```python
from build123d import *

# Parameters (mm, degrees)
SALIENTE_EXTRUIR1_DEPTH = 7
CROQUIS2_R              = 2.5
CORTAR_EXTRUIR1_DEPTH   = 8
CROQUIS3_R              = 1.5
CORTAR_EXTRUIR2_DEPTH   = 8
CROQUIS4_R              = 11
CROQUIS4_R_2            = 2.5
SALIENTE_EXTRUIR2_DEPTH = 2
REDONDEO1_R             = 0.1
REDONDEO3_R             = 0.25


with BuildPart() as part:
    # Croquis1 → Saliente-Extruir1 (new body)
    with BuildSketch(Plane(origin=(0, 0, 0), x_dir=(1, 0, 0), z_dir=(0, 1, 0))):
        Polygon((0, 32.526911935), (2.473088065, 35), (32.526911935, 35), (35, 32.526911935), (35, 2.473088065), (32.526911935, 0), (2.473088065, 0), (0, 2.473088065), align=None)
    extrude(amount=SALIENTE_EXTRUIR1_DEPTH)

    # Croquis2 → Cortar-Extruir1 (cut, through all)
    with BuildSketch(Plane(origin=(0, 7, 0), x_dir=(1, 0, 0), z_dir=(0, 1, 0))):
        with Locations((17.5, 17.5)):
            Circle(CROQUIS2_R)
    extrude(amount=-CORTAR_EXTRUIR1_DEPTH, mode=Mode.SUBTRACT)

    # Croquis3 → Cortar-Extruir2 (cut, through all)
    with BuildSketch(Plane(origin=(0, 7, 0), x_dir=(1, 0, 0), z_dir=(0, 1, 0))):
        with Locations((4.5, 30.5)):
            Circle(CROQUIS3_R)
        with Locations((30.5, 30.5)):
            Circle(CROQUIS3_R)
        with Locations((30.5, 4.5)):
            Circle(CROQUIS3_R)
        with Locations((4.5, 4.5)):
            Circle(CROQUIS3_R)
    extrude(amount=-CORTAR_EXTRUIR2_DEPTH, mode=Mode.SUBTRACT)

    # Croquis4 → Saliente-Extruir2 (add)
    with BuildSketch(Plane(origin=(0, 7, 0), x_dir=(1, 0, 0), z_dir=(0, 1, 0))):
        with Locations((17.5, 17.5)):
            Circle(CROQUIS4_R)
        with Locations((17.5, 17.5)):
            Circle(CROQUIS4_R_2, mode=Mode.SUBTRACT)
    extrude(amount=SALIENTE_EXTRUIR2_DEPTH)

    # Redondeo1
    redondeo1_edges = [part.edges().sort_by_distance(p)[0] for p in [
        (6.5, 9, -17.5),
    ]]
    fillet(redondeo1_edges, radius=REDONDEO1_R)

    # Redondeo3
    redondeo3_edges = [part.edges().sort_by_distance(p)[0] for p in [
        (17.5, 7, 0),
        (33.763455967, 7, -1.236544033),
        (35, 7, -17.5),
        (33.763455967, 7, -33.763455967),
        (17.5, 7, -35),
        (1.236544033, 7, -33.763455967),
        (0, 7, -17.5),
        (1.236544033, 7, -1.236544033),
    ]]
    fillet(redondeo3_edges, radius=REDONDEO3_R)


solid = part.part
```
Can you work these out from the model? Positions are in its coordinate system, mm. A direction names the side the tool comes from. Round coordinates to 2 decimals unless told otherwise and drop trailing zeros. Loops run counter-clockwise (first coordinate to the right, second up) from the corner with the lowest first, then second, coordinate; pieces in that order, holes last. Notation, with made-up numbers: M 40,0 L 69,0 A3 cw 69,5 Z; hole C 86.25,-0.5 d5. An arc over 180 degrees is marked long. Answer as a JSON object with one key per item and string values. Group by question number.
Q1. Will these pins go through, and if not, where does the flat tip stop? pin 1 (4 mm diameter, centred on x = 4.5, z = -30.5, fed in from +Y); pin 2 (1 mm diameter, centred on y = 8, z = -19.5, fed in from +X).
Q2. Imagine slicing it at D-D, the plane x = 30.5. Please give me the cut outline in (y, z), then the cut area to 3 significant figures.
Q3. We'd pull the mould along X, two halves only. Please class faces 1 (the cylindrical face through (33.73, 6.93, -33.69)), 2 (the cylindrical face through (5.886, 3.549, -3.925)), 3 (the flat face through (1.254, 3.328, -1.219)): +X half, -X half, draft (parallel to the pull), parting line (faces both ways), or undercut.
Q4. Imagine slicing it at B-B, the plane x = 17.5. Please give me the cut outline in (y, z).
Q5. Imagine slicing it at C-C, the plane z = -4.5. Please give me the cut outline in (x, y).
Q6. On a 3-axis mill with a long thin cutter (end or side, diameter ignored), from which of +Z, -Z, +X, -X, +Y, -Y can I reach the whole of each face in a straight line? I mean faces 4 (the cylindrical face through (1.31, 6.93, -33.73)), 5 (the cylindrical face through (22.576, 7.937, -7.741)). Say none if no direction works.
Q7. Imagine slicing it at A-A, the plane z = -17.5. Please give me the cut outline in (x, y), then the cut area to 3 significant figures.
Q8. Please list where these lines run through material, in increasing order: L1, parallel to Z at x = 4.5, y = 1.75; L2, parallel to X at y = 5, z = -30.5; L3, parallel to X at y = 8.45, z = -17.5.
Findings:
{
 "1": {"pin 1": "stops at y = 7", "pin 2": "stops at x = 28.4"},
 "2": {"outline": "M 0,-35 L 6.75,-35 A0.25 ccw 7,-34.75 L 7,-32 L 0,-32 Z; M 0,-29 L 7,-29 L 7,-6 L 0,-6 Z; M 0,-3 L 7,-3 L 7,-0.25 A0.25 ccw 6.75,0 L 0,0 Z", "area": "203 mm2"},
 "3": {"face 1": "+X half", "face 2": "undercut", "face 3": "-X half"},
 "4": {"outline": "M 0,-35 L 6.75,-35 A0.25 ccw 7,-34.75 L 7,-28.5 L 8.9,-28.5 A0.1 ccw 9,-28.4 L 9,-20 L 0,-20 Z; M 0,-15 L 9,-15 L 9,-6.6 A0.1 ccw 8.9,-6.5 L 7,-6.5 L 7,-0.25 A0.25 ccw 6.75,0 L 0,0 Z"},
 "5": {"outline": "M 0,0 L 3,0 L 3,7 L 0.25,7 A0.25 ccw 0,6.75 Z; M 6,0 L 29,0 L 29,7 L 6,7 Z; M 32,0 L 35,0 L 35,6.75 A0.25 ccw 34.75,7 L 32,7 Z"},
 "6": {"face 4": "-Z, -X, +Y", "face 5": "+Y"},
 "7": {"outline": "M 0,0 L 15,0 L 15,9 L 6.6,9 A0.1 ccw 6.5,8.9 L 6.5,7 L 0.25,7 A0.25 ccw 0,6.75 Z; M 20,0 L 35,0 L 35,6.75 A0.25 ccw 34.75,7 L 28.5,7 L 28.5,8.9 A0.1 ccw 28.4,9 L 20,9 Z", "area": "244 mm2"},
 "8": {"L1": "z = -35 to -32, -29 to -6, -3 to 0", "L2": "x = 0 to 3, 6 to 29, 32 to 35", "L3": "x = 6.5 to 15, 20 to 28.5"}
}
